Could you check a few things on this model? Use its own coordinates, in mm. A direction names the side the tool comes from. Round coordinates to 2 decimals unless told otherwise and drop trailing zeros. Loops run counter-clockwise (first coordinate to the right, second up) from the corner with the lowest first, then second, coordinate; pieces in that order, holes last. Notation, with made-up numbers: (-31.5, 30) -> (12.5, 30) arc R37 ccw to (12.5, 68) -> close; hole circle Ø7 at (71, -28.75). An arc over 180 degrees is marked (long way). Put each result on its own line as item: value. Start each with the question number.
1. Imagine slicing it at C-C, the plane x = 11. Please give me the cut outline in (y, z).
2. Imagine slicing it at B-B, the plane z = 11. Please give me the cut outline in (x, y), and give its area (3 significant figures).
3. Which directions (+Z, -Z, +X, -X, +Y, -Y) give clear straight access to the entire face, cutting with the end or side of a thin tool? Please do faces 4 (the flat face through (9.114, -0.112, 9.629)), 5 (the flat face through (13, 12, 7)), 6 (the flat face through (3.904, -0.112, 6.742)).
4. If we mould it in two halves opening along X, with no side actions, what happens to faces 1 (the cylindrical face through (-1.5, -9.97, 0.07)), 2 (the cylindrical face through (-3.22, 9.97, -1.37)), 3 (the flat face through (22.877, -10.028, 10.436))? For each: pulls with the +X half, pulls with the -X half, needs draft (parallel to the pull), parting line crosses it, or undercut.
5. I'm going to push flat-ended pins straight in: P1, Ø1.8, axis at x = 18.7, z = 20.706, coming from the -Y side; P2, Ø8, axis at y = 6, z = 6.5, coming from the +X side; P3, Ø12, axis at y = 2.5, z = 16.5, coming from the +X side; P4, Ø4, axis at x = 4.5, y = -5, coming from the +Z side. Where does each tip first touch, or does it pass through?
6. I need wall thicknesses on line 1 (X direction, y = 10.9, z = 0); line 2 (Y direction, x = -2, z = 1); line 3 (Z direction, x = 18.7, y = -11.1). Which ranges of each line are inside material? Lowest first, please. Write a range as [from, to].
7. Imagine slicing it at A-A, the plane x = 1. Please give me the cut outline in (y, z), and give its area (3 significant figures).
8. Imagine slicing it at D-D, the plane y = -4.5. Please give me the cut outline in (x, z).
```python
from build123d import *

# Parameters (mm, degrees)
F0_R     = 1.5
F1_DEPTH = 12
F4_DEPTH = 8
F5_DEPTH = 8


with BuildPart() as f1:
    # F0 (on Front) → F1 (new body, symmetric)
    with BuildSketch(Plane.XZ):
        with BuildLine():
            Line((16.1025038779, 23.0518503566), (-2.5974961221, 2.3458503566))
            ThreePointArc((-2.5974961221, 2.3458503566), (-3.1984743432, -1.4211832661), (0, -3.5))
            Line((0, -3.5), (20.05, -3.5))
            ThreePointArc((20.05, -3.5), (22.6041132903, -2.3930117635), (23.5425846566, 0.2277112569))
            Line((23.5425846566, 0.2277112569), (22.1925846566, 20.9337112569))
            ThreePointArc((22.1925846566, 20.9337112569), (19.8497496173, 24.0117640293), (16.1025038779, 23.0518503566))
        make_face()
        Circle(F0_R, mode=Mode.SUBTRACT)
        with Locations((20.05, 0)):
            Circle(F0_R, mode=Mode.SUBTRACT)
        with Locations((18.7, 20.706)):
            Circle(F0_R, mode=Mode.SUBTRACT)
    extrude(amount=F1_DEPTH, both=True)

    # F3 (on Front) → F4 (cut, symmetric)
    with BuildSketch(Plane.XZ):
        with BuildLine():
            ThreePointArc((-2.5974961221, 2.3458503566), (-3.1984743432, -1.4211832661), (0, -3.5))
            Line((0, -3.5), (20.05, -3.5))
            ThreePointArc((20.05, -3.5), (22.6041132903, -2.3930117635), (23.5425846566, 0.2277112569))
            Line((23.5425846566, 0.2277112569), (22.1925846566, 20.9337112569))
            ThreePointArc((22.1925846566, 20.9337112569), (19.8497496173, 24.0117640293), (16.1025038779, 23.0518503566))
            Line((16.1025038779, 23.0518503566), (-2.5974961221, 2.3458503566))
        make_face()
    extrude(amount=F4_DEPTH, both=True, mode=Mode.SUBTRACT)

    # F2 (on Front) → F5 (join, symmetric)
    with BuildSketch(Plane.XZ):
        Polygon((10.1706322474, 16.4836506784), (2.5097552257, 8.0009704853), (5.33731529, 5.4473448114), (12.9981923117, 13.9300250045), align=None)
    extrude(amount=F5_DEPTH, both=True)


solid = f1.part
```
Entries:
1. outline: (-12, -3.5) -> (-8, -3.5) -> (-8, 11.72) -> (8, 11.72) -> (8, -3.5) -> (12, -3.5) -> (12, 17.4) -> (8, 17.4) -> (8, 15.73) -> (-8, 15.73) -> (-8, 17.4) -> (-12, 17.4) -> close
2. outline: (5.22, -12) -> (22.84, -12) -> (22.84, -8) -> (10.35, -8) -> (10.35, 8) -> (22.84, 8) -> (22.84, 12) -> (5.22, 12) -> close
2. area: 223 mm^2
3. face 4: -Z, +X
3. face 5: +Z, -Z, +X, -X, +Y
3. face 6: -Z, -X
4. face 1: undercut
4. face 2: pulls with the -X half
4. face 3: pulls with the +X half
5. P1: through
5. P2: x = 23.36
5. P3: x = 22.64
5. P4: z = 12.42
6. line 1: [-3.5, -1.5], [1.5, 18.55], [21.55, 23.55]
6. line 2: [-12, -8], [8, 12]
6. line 3: [-3.5, -0.65], [0.65, 19.21], [22.21, 24.21]
7. outline: (-12, -3.5) -> (-8, -3.5) -> (-8, -1.12) -> (-12, -1.12) -> close; (-12, 1.12) -> (-8, 1.12) -> (-8, 6.33) -> (-12, 6.33) -> close; (8, -3.5) -> (12, -3.5) -> (12, -1.12) -> (8, -1.12) -> close; (8, 1.12) -> (12, 1.12) -> (12, 6.33) -> (8, 6.33) -> close
7. area: 60.7 mm^2
8. outline: (2.51, 8) -> (5.34, 5.45) -> (13, 13.93) -> (10.17, 16.48) -> close
